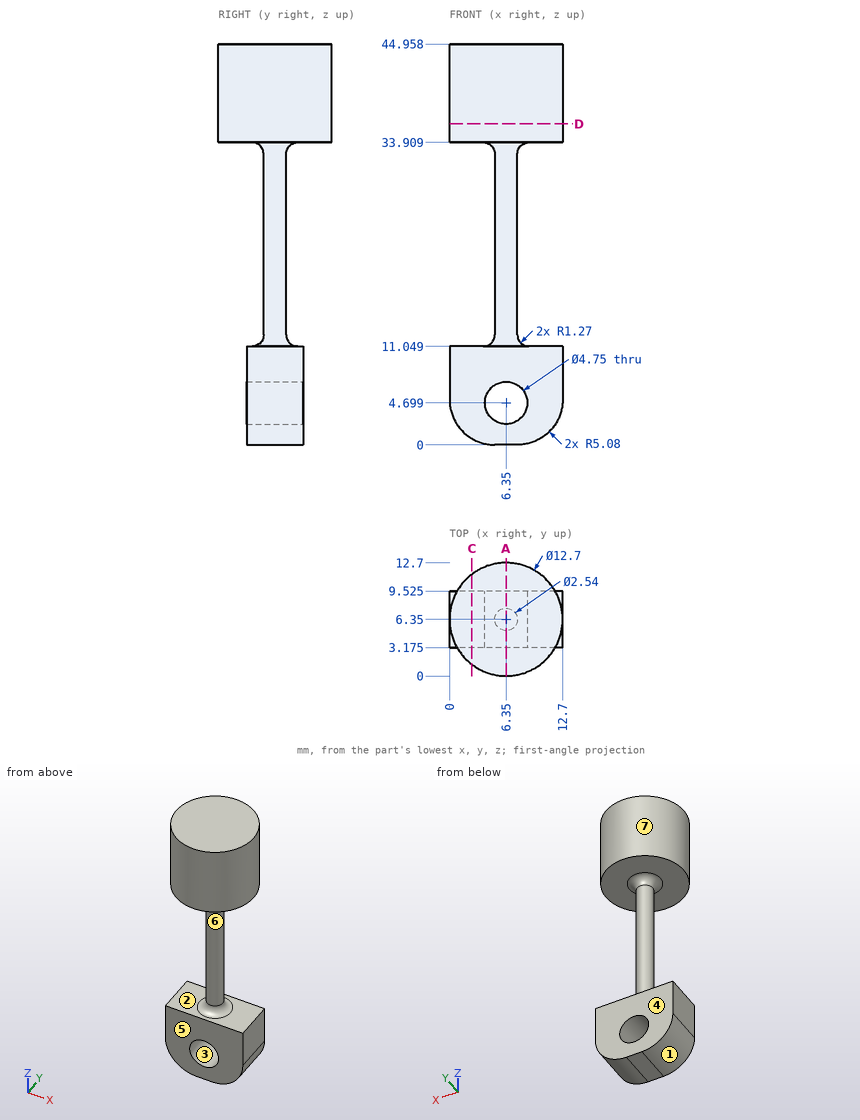
Study the drawing (mm; zero at the part's minimum x, y, z) and answer. A direction names the side the tool comes from. Round coordinates to 2 decimals unless told otherwise and drop trailing zeros. Loops run counter-clockwise (first coordinate to the right, second up) from the corner with the lowest first, then second, coordinate; pieces in that order, holes last. Notation, with made-up numbers: (-6, 57.25) - (13, 57.25) arc R25 ccw to (13, 89.25) - close; hole circle Ø2 at (34.25, 2.5). An arc over 180 degrees is marked (long way). Use one line per item in the form item = value. Start each with the question number.
1. The part is cut by section D-D on z = 36. Determine the outline of the cut face in (x, y).
2. A tool of negligible diameter and unlimited length cuts with its end or side. For the marked faces 4, 5, 6 and 7, from which of +Z, -Z, +X, -X, +Y, -Y can it reach the whole face along a straight path? Write none if from no direction.
3. For a pull along X with two mould halves and no side action, classify the marked faces 1, 2 and 3 as pulls with the +X half, pulls with the -X half, needs draft (parallel to the pull), parting line crosses it, or undercut.
4. Given pin 1 Ø5 at (y, z) = (4.5, 28.5) entering from -X; pin 2 Ø5.5 at (x, z) = (6.35, 4.699) entering from -Y (3 decimals); pin 3 Ø5 at (x, z) = (6.5, 13) entering from +Y (3 decimals), each flat-ended and moving along its own axis, determine where each tip first touches the part or whether it passes through.
5. The part is cut by section C-C on x = 2.5. Determine the outline of the cut face in (y, z) (1 decimal).
6. The part is cut by section A-A on x = 6.35. Determine the outline of the cut face in (y, z) (1 decimal).
7. Consider line 1 (Z direction, x = 7.5, y = 9.25); line 2 (Z direction, x = 6.35, y = 7.25); line 3 (Z direction, x = 7.5, y = 4.75). Determine where each line is inside the solid, lowest interval first. Write a range as [from, to].
Geometry check:
q1.outline = circle Ø12.7 at (6.35, 6.35)
q2.face_4 = -Z, +X, -X, +Y
q2.face_5 = -Z, +X, -X, -Y
q2.face_6 = none
q2.face_7 = +Z
q3.face_1 = pulls with the -X half
q3.face_2 = needs draft
q3.face_3 = undercut
q4.pin_1 = 5.08
q4.pin_2 = 3.175
q4.pin_3 = 9.525
q5.outline = (1.3, 33.9) - (11.4, 33.9) - (11.4, 45) - (1.3, 45) - close; (3.2, 0.7) - (9.5, 0.7) - (9.5, 11) - (3.2, 11) - close
q6.outline = (0, 33.9) - (3.8, 33.9) arc R1.3 cw to (5.1, 32.6) - (5.1, 12.3) arc R1.3 cw to (3.8, 11) - (3.2, 11) - (3.2, 7.1) - (9.5, 7.1) - (9.5, 11) - (8.9, 11) arc R1.3 cw to (7.6, 12.3) - (7.6, 32.6) arc R1.3 cw to (8.9, 33.9) - (12.7, 33.9) - (12.7, 45) - (0, 45) - close; (3.2, 0) - (9.5, 0) - (9.5, 2.3) - (3.2, 2.3) - close
q7.line_1 = [0, 2.62], [6.78, 11.05], [33.91, 44.96]
q7.line_2 = [0, 2.32], [7.07, 44.96]
q7.line_3 = [0, 2.62], [6.78, 11.18], [33.77, 44.96]
